The listing builds one solid part. Answer for the finished solid, in the listing's coordinates (mm). A direction names the side the tool comes from. Coordinates: 2 decimals unless noted, no trailing zeros. Write each loop counter-clockwise with the first axis right and the second up, starting at its lowest first coordinate (ties: lowest second). Pieces come first, ordered by that corner, then holes. Notation, with made-up numbers: M 80.25,7 L 132.25,7 A21 ccw 132.25,29 Z; hole C 14,34.25 d4. An arc over 180 degrees is marked long. Answer as CSV lines item,"result".
```python
from build123d import *

# Parameters (mm, degrees)
F0_W     = 229.108
F0_H     = 151.8412
F1_DEPTH = 3.175
F2_W     = 216.154
F2_H     = 137.8712
F3_DEPTH = 0.254
F4_W     = 44.7675
F4_H     = 27.94
F5_DEPTH = 2.54
F7_DEPTH = 3.81
F8_R     = 3.80999


# Not quite as in the source:
# - a fillet or chamfer is up to 0.001 mm smaller than in the source, because OpenCascade refuses the exact size


with BuildPart() as f1:
    # F0 (on Front) → F1 (new body)
    with BuildSketch(Plane.XZ):
        with Locations((114.554, 75.9206)):
            Rectangle(F0_W, F0_H)
    extrude(amount=F1_DEPTH)

    # F2 (on face) → F3 (cut)
    with BuildSketch(Plane.XZ.offset(3.175)):
        with Locations((114.046, 77.1906)):
            Rectangle(F2_W, F2_H)
    extrude(amount=-F3_DEPTH, mode=Mode.SUBTRACT)

    # F4 (on face) → F5 (join)
    with BuildSketch(Plane(origin=(0, 0, 0), x_dir=(-1, 0, 0), z_dir=(0, 1, 0))):
        with Locations((-191.16675, 16.51)):
            Rectangle(F4_W, F4_H)
    extrude(amount=F5_DEPTH)

    # F6 (on face) → F7 (join)
    with BuildSketch(Plane(origin=(0, 2.54, 0), x_dir=(-1, 0, 0), z_dir=(0, 1, 0))):
        Polygon((-210.21675, 30.48), (-210.21675, 24.13), (-172.11675, 24.13), (-172.11675, 30.48), (-191.16675, 49.53), align=None)
    extrude(amount=F7_DEPTH)

    # F8 (radius 3.81 in the source; OpenCascade refuses exactly that, so slightly less here)
    f8_edges = [f1.edges().sort_by_distance(p)[0] for p in [
        (200.69175, 6.35, 40.005),
        (181.64175, 6.35, 40.005),
    ]]
    fillet(f8_edges, radius=F8_R)


solid = f1.part
```
Q1. Find section B-B (x = 153.5). Give the vertices of the cut face in (y, z) (3 decimals), and give its area (3 significant figures).
Output:
outline,"M -3.175,0 L 0,0 L 0,151.841 L -3.175,151.841 L -3.175,146.126 L -2.921,146.126 L -2.921,8.255 L -3.175,8.255 Z"
area,"447 mm2"
Q2. Flat-ended cylindrical pins translate along their axes: pin 1 Ø4 at (y, z) = (3.5, 27) entering from -X; pin 2 Ø0.8 at (y, z) = (1.5, 11) entering from +X; pin 3 Ø5.5 at (x, z) = (197.5, 42) entering from -Y; pin 4 Ø4 at (y, z) = (2.5, 105) entering from +X. Find the tip coordinate at first contact, or state that the pin passes through.
Output:
pin 1,"x = 168.78"
pin 2,"x = 213.55"
pin 3,"y = -2.92"
pin 4,"through"
Q3. Straight lines are drawn through the part: line 1 (Y direction, x = 150.5, z = 26); line 2 (X direction, y = 1, z = 18.5); line 3 (Z direction, x = 202, y = 1.25). For each, find the intervals that lie inside material, in ascending order.
Output:
line 1,"-2.92 to 0"
line 2,"168.78 to 213.55"
line 3,"2.54 to 30.48"
Q4. Find section A-A (z = 113). Give the vertices of the cut face in (x, y) (3 decimals), and give its area (3 significant figures).
Output:
outline,"M 0,-3.175 L 5.969,-3.175 L 5.969,-2.921 L 222.123,-2.921 L 222.123,-3.175 L 229.108,-3.175 L 229.108,0 L 0,0 Z"
area,"673 mm2"
Q5. The mould has two halves that part along X. Classify faces 1 (the flat face through (113, 0, 77)), 2 (the cylindrical face through (201.423, 5.204, 37.738)), 3 (the flat face through (113, -2.921, 78)): pulls with the +X half, pulls with the -X half, needs draft (parallel to the pull), parting line crosses it, or undercut.
Output:
face 1,"needs draft"
face 2,"pulls with the +X half"
face 3,"undercut"
Q6. Find section C-C (y = 4.5). Give the vertices of the cut face in (x, z).
Output:
outline,"M 172.12,24.13 L 210.22,24.13 L 210.22,29.71 L 191.17,48.76 L 172.12,29.71 Z"
Q7. For faces 4 (the flat face through (191, 6.35, 32)), 5 (the flat face through (191, 2.54, 38)), determine the directions among +Z, -Z, +X, -X, +Y, -Y from which every point of the face is accessible in a straight line to the end or side of a thin tool.
Output:
face 4,"+Z, -Z, +X, -X, +Y"
face 5,"+Z, +X, -X"
